```python
from build123d import *

# Parameters (mm, degrees)
SKETCH1_W             = 60
SKETCH1_H             = 8
BOSS_EXTRUDE1_DEPTH   = 4
SKETCH3_W             = 95
SKETCH3_H             = 70
SKETCH3_R             = 1.38
BOSS_EXTRUDE2_DEPTH   = 2
FILLET3_R             = 2
F_3_0MM_DOWEL_HOLE2_D = 3


with BuildPart() as part:
    # Sketch1 → Boss-Extrude1 (new body)
    with BuildSketch(Plane(origin=(0, 0, 0), x_dir=(1, 0, 0), z_dir=(0, 1, 0))):
        with Locations((30, 4)):
            Rectangle(SKETCH1_W, SKETCH1_H)
    extrude(amount=BOSS_EXTRUDE1_DEPTH)

    # Sketch3 → Boss-Extrude2 (add)
    with BuildSketch(Plane(origin=(0, 0, -8), x_dir=(-1, 0, 0), z_dir=(0, 0, -1))):
        with Locations((-30, 39)):
            Rectangle(SKETCH3_W, SKETCH3_H)
        with Locations((13, 68)):
            Circle(SKETCH3_R, mode=Mode.SUBTRACT)
        with Locations((-73, 68)):
            Circle(SKETCH3_R, mode=Mode.SUBTRACT)
        with Locations((-73, 10)):
            Circle(SKETCH3_R, mode=Mode.SUBTRACT)
        with Locations((13, 10)):
            Circle(SKETCH3_R, mode=Mode.SUBTRACT)
        Polygon((-3.5, 10), (7.5, 65), (7.5, 10), align=None, mode=Mode.SUBTRACT)
        Polygon((-16.5, 10), (-5.5, 10), (-16.5, 65), align=None, mode=Mode.SUBTRACT)
        Polygon((-18, 10), (-29, 10), (-18, 65), align=None, mode=Mode.SUBTRACT)
        Polygon((-42, 10), (-31, 10), (-42, 65), align=None, mode=Mode.SUBTRACT)
        Polygon((-43.5, 10), (-54.5, 10), (-43.5, 65), align=None, mode=Mode.SUBTRACT)
        Polygon((-67.5, 10), (-56.5, 10), (-67.5, 65), align=None, mode=Mode.SUBTRACT)
    extrude(amount=-BOSS_EXTRUDE2_DEPTH)

    # Fillet3
    fillet3_edges = [part.edges().sort_by_distance(p)[0] for p in [
        (30, 4, -6),
    ]]
    fillet(fillet3_edges, radius=FILLET3_R)

    # Ø3.0mm Dowel Hole2 (through all)
    with Locations(Plane(origin=(0, 74, 0), x_dir=(1, 0, 0), z_dir=(0, 1, 0))):
        with Locations((10, 3), (30, 3), (50, 3)):
            Hole(F_3_0MM_DOWEL_HOLE2_D / 2)


solid = part.part
```
The model under review builds one solid part; all positions refer to its coordinate system, in mm. A direction names the side the tool comes from. Round coordinates to 2 decimals unless told otherwise and drop trailing zeros. Write each loop counter-clockwise with the first axis right and the second up, starting at its lowest first coordinate (ties: lowest second). Pieces come first, ordered by that corner, then holes. Notation, with made-up numbers: (38, 27.25) - (50, 27.25) arc R12 cw to (50, 44.25) - close; hole circle Ø3 at (-37, 85.25). An arc over 180 degrees is marked (long way). One line per question, with ' | ' between items.
Item 1: Add section C-C, the plane z = -3. Give the boundary of the cut face in (x, y), then the cut area to 3 significant figures.
Resolved:
outline: (0, 0) - (8.5, 0) - (8.5, 4) - (0, 4) - close; (11.5, 0) - (28.5, 0) - (28.5, 4) - (11.5, 4) - close; (31.5, 0) - (48.5, 0) - (48.5, 4) - (31.5, 4) - close; (51.5, 0) - (60, 0) - (60, 4) - (51.5, 4) - close | area: 204 mm2
Item 2: For faces 5 (the face through (11, 10, -7)), 6 (the face through (-17.5, 39, -7)), list the 3-axis set-ups (+Z, -Z, +X, -X, +Y, -Y) from which the entire face can be reached by the end or side of a thin tool; tool diameter is ignored.
Resolved:
face 5: +Z, -Z | face 6: +Z, -Z, -X, +Y, -Y
Item 3: To check wall thickness, follow probe 1 along Y at (x, z) = (-13, -6.6); probe 2 along X at (y, z) = (68, -7.6); probe 3 along Z at (x, y) = (30, 0.8). State the ranges of each line that lie inside material, in increasing order.
Resolved:
probe 1: y = 4 to 8.62, 11.38 to 66.62, 69.38 to 74 | probe 2: x = -17.5 to -14.38, -11.62 to 71.62, 74.38 to 77.5 | probe 3: z = -8 to -4.5, -1.5 to 0
Item 4: For P1, Ø4.5, axis at x = -13, y = 68, coming from the +Z side; P2, Ø1, axis at x = -5.5, z = -7, coming from the -Y side; P3, Ø4.5, axis at x = 37.5, z = -1.5, coming from the +Y side; P4, Ø1.7, axis at x = 73, y = 68, coming from the -Z side, all flat-tipped, find the tip position at first contact; note any pin that passes through.
Resolved:
P1: stops at z = -6 | P2: stops at y = 4 | P3: stops at y = 4 | P4: passes through
Item 5: The part is to be moulded in two halves that separate along X. For faces 1 (the face through (77.5, 39, -7)), 2 (the face through (30, 2, 0)), 3 (the face through (-1.923, 37.115, -7.014)), 4 (the face through (23.577, 37.115, -7.014)), say which applies: pulls with the +X half, pulls with the -X half, needs draft (parallel to the pull), parting line crosses it, or undercut.
Resolved:
face 1: pulls with the +X half | face 2: needs draft | face 3: undercut | face 4: undercut
Item 6: Add section B-B, the plane y = 30. Give the boundary of the cut face in (x, z), then the cut area to 3 significant figures.
Resolved:
outline: (-17.5, -8) - (-7.5, -8) - (-7.5, -6) - (-17.5, -6) - close; (-0.5, -8) - (9.5, -8) - (9.5, -6) - (-0.5, -6) - close; (16.5, -8) - (18, -8) - (18, -6) - (16.5, -6) - close; (25, -8) - (35, -8) - (35, -6) - (25, -6) - close; (42, -8) - (43.5, -8) - (43.5, -6) - (42, -6) - close; (50.5, -8) - (60.5, -8) - (60.5, -6) - (50.5, -6) - close; (67.5, -8) - (77.5, -8) - (77.5, -6) - (67.5, -6) - close | area: 106 mm2
Item 7: Add section D-D, the plane x = -4. Give the boundary of the cut face in (y, z), then the cut area to 3 significant figures.
Resolved:
outline: (4, -8) - (10, -8) - (10, -6) - (4, -6) - close; (47.5, -8) - (74, -8) - (74, -6) - (47.5, -6) - close | area: 65.0 mm2
Item 8: Add section A-A, the plane x = 10. Give the boundary of the cut face in (y, z), then the cut area to 3 significant figures.
Resolved:
outline: (0, -8) - (10, -8) - (10, -6) - (6, -6) arc R2 cw to (4.06, -4.5) - (0, -4.5) - close; (0, -1.5) - (4, -1.5) - (4, 0) - (0, 0) - close; (32.5, -8) - (74, -8) - (74, -6) - (32.5, -6) - close | area: 116 mm2
